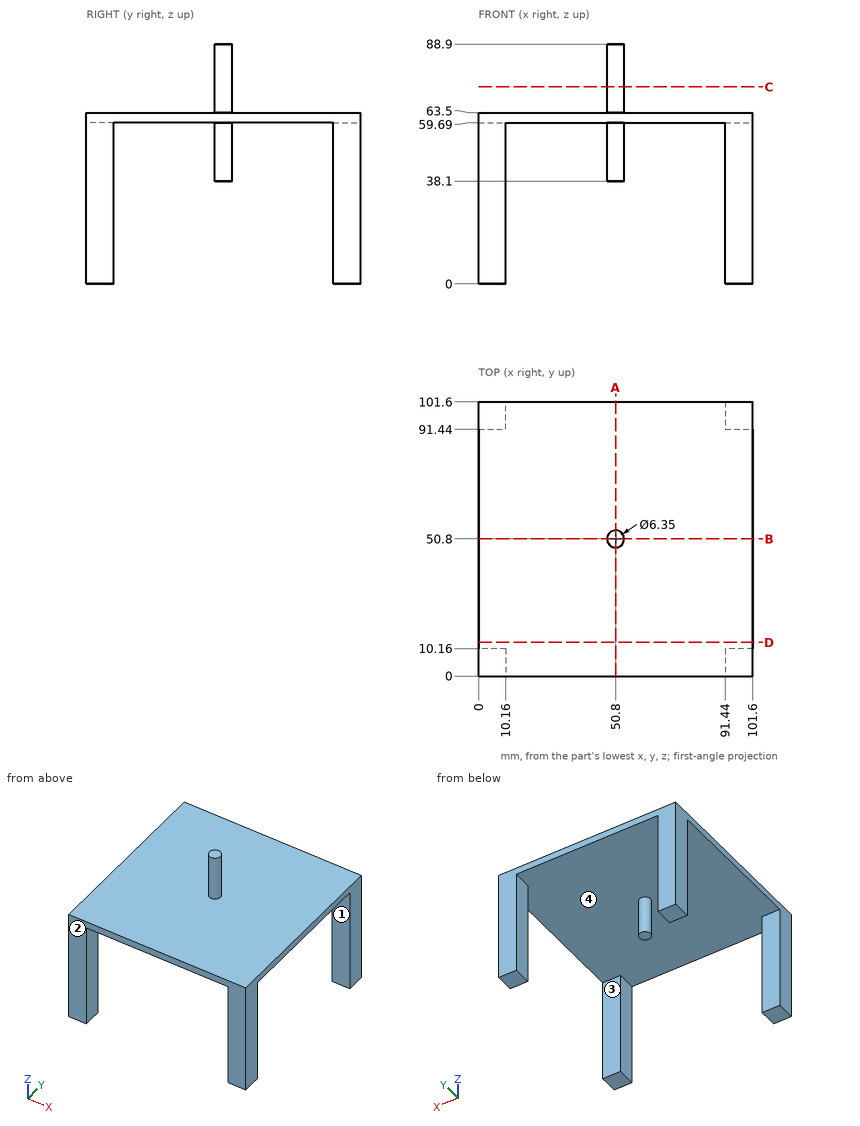
The figure shows three views and two pictorial views of one solid part (mm, origin at its lowest corner). Answer the questions. A direction names the side the tool comes from. Coordinates: 2 decimals unless noted, no trailing zeros. Order: outer loops, then holes, each group sorted by start corner. A loop starts at its lowest first (then second) coordinate and runs counter-clockwise, first axis right, second up. Notation, with made-up numbers: M 66.25,13.25 L 102.25,13.25 A10 cw 102.25,20.25 Z; hole C 13.5,-31.5 d1. An arc over 180 degrees is marked long. Use CSV: the item, a comma, the result in double quotes.
1) Section D-D on y = 12.5 is taken. Write down the section's boundary in (x, z).
Worked out:
outline,"M 0,59.69 L 101.6,59.69 L 101.6,63.5 L 0,63.5 Z"
2) Section C-C on z = 73 is taken. Write down the section's boundary in (x, y) (3 decimals).
Worked out:
outline,"C 50.8,50.8 d6.35"
3) For the marked faces 1 and 2, determine the directions among +Z, -Z, +X, -X, +Y, -Y from which every point of the face is accessible in a straight line to the end or side of a thin tool.
Worked out:
face 1,"-Z, +X, -X"
face 2,"+Z, -Z, +X, -X, -Y"
4) Determine the mould class of the marked faces 3 and 4 for opening direction X: released by +X, released by -X, zero draft, split by the parting line, or undercut.
Worked out:
face 3,"zero draft"
face 4,"undercut"
5) Section A-A on x = 50.8 is taken. Write down the section's boundary in (y, z) (3 decimals), plus the area to 3 significant figures.
Worked out:
outline,"M 0,59.69 L 47.625,59.69 L 47.625,38.1 L 53.975,38.1 L 53.975,59.69 L 101.6,59.69 L 101.6,63.5 L 53.975,63.5 L 53.975,88.9 L 47.625,88.9 L 47.625,63.5 L 0,63.5 Z"
area,"685 mm^2"
6) Flat-ended cylindrical pins translate along their axes: pin 1 Ø2 at (x, y) = (60, 63) entering from +Z; pin 2 Ø1.5 at (x, y) = (63, 27) entering from -Z; pin 3 Ø11 at (y, z) = (96, 15) entering from -X; pin 4 Ø1.9 at (x, y) = (52.5, 51.5) entering from -Z. Find the tip coordinate at first contact, or state that the pin passes through.
Worked out:
pin 1,"stops at z = 63.5"
pin 2,"stops at z = 59.69"
pin 3,"stops at x = 0"
pin 4,"stops at z = 38.1"
7) Consider line 1 (Z direction, x = 86, y = 58); line 2 (Z direction, x = 8, y = 9). Determine where each line is inside the solid, lowest interval first. Write a range as [from, to].
Worked out:
line 1,"z = [59.69, 63.5]"
line 2,"z = [0, 63.5]"
